Input: part model. Units: mm. Frame: model coordinates. A direction names the side the tool comes from. Give positions to 0.01 mm unless a question says otherwise; leave off trailing zeros. Write each loop counter-clockwise with the first axis right and the second up, starting at its lowest first coordinate (ties: lowest second). Pieces come first, ordered by that corner, then holes. Notation, with made-up numbers: (79.5, 70) -> (114.5, 70) arc R25 cw to (114.5, 91) -> close; hole circle Ø11 at (9.5, -14). An arc over 180 degrees is marked (long way). Return JSON: item names as keys, results as strings. Group by question number.
Item 1: Section B-B, the plane z = 0. Return loops of the section in (x, y), then the cut area to 3 significant figures.
Item 2: Section A-A, the plane x = 0. Return loops of the section in (y, z).
Item 3: Pin query (flat end, axial travel): P1, Ø2, axis at x = 1.5, y = 5, coming from the +Z side; P2, Ø4, axis at x = -3, z = 4, coming from the +Y side; P3, Ø1, axis at y = 11, z = 1.5, coming from the -X side. Return the tip coordinate at first contact, or that it passes through.
Item 4: Section C-C, the plane y = 4.25. Return loops of the section in (x, z).
Item 5: Section D-D, the plane y = 11. Return loops of the section in (x, z), then the cut area to 3 significant figures.
Item 6: Mould query, pull axis X, two halves, no side actions, for faces 1 (the face through (1, 11, 0)), 2 (the face through (0, 10, 0)), 3 (the face through (3.3, 8, -0.1)), 4 (the face through (4.88, 9.01, 1.08)). Classes: released by +X, released by -X, zero draft, split by the parting line, or undercut.
Item 7: Line query: line 1 (Z direction, x = -1, y = 8.75); line 2 (X direction, y = 10.25, z = 4); line 3 (Y direction, x = 0.5, z = 1.75). Output: solid intervals per line, ascending. Write a range as [from, to].
Item 8: Set-up query: faces 5 (the face through (-1, 11, 0)), 6 (the face through (0, 0, 0)), 7 (the face through (-0.9, 4.55, -2.86)). Return all of +Z, -Z, +X, -X, +Y, -Y with unobstructed straight access to the full face (end or side cutting, diameter ignored); none if empty.
from build123d import *

# Parameters (mm, degrees)
DOME4_FACE_RADIUS = 5
DOME4_HEIGHT      = 2
SKETCH3_W         = 2
SKETCH3_H         = 11.201368044
EXTRUDE3_DEPTH    = 2


with BuildPart() as part:
    # Sketch1 → Revolve3 (revolve)
    with BuildSketch(Plane.XY, mode=Mode.PRIVATE) as revolve3_sk:
        Polygon((0, 0), (-2, 0), (-2, 1), (-3, 1), (-3, 8), (-5, 8), (-5, 10), (0, 10), align=None)
    revolve(revolve3_sk.sketch.rotate(Axis((0, 0, 0), (0, 1, 0)), 270), axis=Axis((0, 0, 0), (0, 1, 0)))

    # Dome4: a dome of height H over a round flat face of radius A is a cap of a sphere of radius (A * A + H * H) / (2 * H)
    dome4_r = (DOME4_FACE_RADIUS * DOME4_FACE_RADIUS + DOME4_HEIGHT * DOME4_HEIGHT) / (2 * DOME4_HEIGHT)
    dome4_base = Plane((0, 10, 0), z_dir=(0, 1, 0))
    with Locations(dome4_base.offset(DOME4_HEIGHT - dome4_r)):
        dome4_ball = Sphere(dome4_r, mode=Mode.PRIVATE)
    add(split(dome4_ball, bisect_by=dome4_base, keep=Keep.TOP, mode=Mode.PRIVATE))

    # Sketch3 → Extrude3 (cut)
    with BuildSketch(Plane(origin=(0, 10, 0), x_dir=(1, 0, 0), z_dir=(0, 1, 0))):
        Rectangle(SKETCH3_W, SKETCH3_H)
    extrude(amount=EXTRUDE3_DEPTH, mode=Mode.SUBTRACT)


solid = part.part
Answer below:
{
 "1": {"outline": "(-5, 8) -> (-3, 8) -> (-3, 1) -> (-2, 1) -> (-2, 0) -> (2, 0) -> (2, 1) -> (3, 1) -> (3, 8) -> (5, 8) -> (5, 10) arc R7.25 ccw to (1, 11.93) -> (1, 10) -> (-1, 10) -> (-1, 11.93) arc R7.25 ccw to (-5, 10) -> close", "area": "75.8 mm2"},
 "2": {"outline": "(0, -2) -> (1, -2) -> (1, -3) -> (8, -3) -> (8, -5) -> (10, -5) -> (10, 5) -> (8, 5) -> (8, 3) -> (1, 3) -> (1, 2) -> (0, 2) -> close"},
 "3": {"P1": "stops at z = 2.96", "P2": "stops at y = 11.35", "P3": "stops at x = -4.17"},
 "4": {"outline": "circle Ø6 at (0, 0)"},
 "5": {"outline": "(-1, -3.54) -> (-1, 3.54) arc R3.67 ccw to start; (1, -3.54) arc R3.67 ccw to (1, 3.54) -> close", "area": "27.9 mm2"},
 "6": {"face 1": "undercut", "face 2": "undercut", "face 3": "zero draft", "face 4": "split by the parting line"},
 "7": {"line 1": "z = [-4.9, 4.9]", "line 2": "x = [-2.51, -1], [1, 2.51]", "line 3": "y = [0, 10]"},
 "8": {"face 5": "+Z, -Z, +Y", "face 6": "+Z, -Z, +X, -X, -Y", "face 7": "-Y"}
}
